Check sheet for the modelled part. Datum: model origin and axes. Units: mm. A direction names the side the tool comes from. Coordinates: 2 decimals unless noted, no trailing zeros. Loops run counter-clockwise (first coordinate to the right, second up) from the corner with the lowest first, then second, coordinate; pieces in that order, holes last. Notation, with made-up numbers: M -29,66 L 16,66 A33 ccw 16,104 Z; hole C 6,-7.5 d11. An arc over 180 degrees is marked long. Return JSON: item names as keys, results as strings.
from build123d import *

# Parameters (mm, degrees)
SKETCH1_W                = 63
SKETCH1_H                = 53
BOSS_EXTRUDE1_DEPTH      = 2
SKETCH2_W                = 15.24
SKETCH2_H                = 10.16
CUT_EXTRUDE1_DEPTH       = 1
BOSS_EXTRUDE2_DEPTH      = 0.1
BOSS_EXTRUDE2_DEPTH_BACK = 2.1
SKETCH4_R                = 2
SKETCH4_R_2              = 1
SKETCH4_W                = 5.013644296
SKETCH4_H                = 5.037668264
SKETCH4_W_2              = 4.110148076
SKETCH4_H_2              = 4.160405132
CUT_EXTRUDE2_START       = -2
SKETCH5_R                = 1
CUT_EXTRUDE2_DEPTH       = 2
EXTRUDE_THIN1_DEPTH      = 0.5
EXTRUDE_THIN1_DEPTH_BACK = 0.5
FILLET1_R                = 0.25


with BuildPart() as part:
    # Sketch1 → Boss-Extrude1 (new body)
    with BuildSketch(Plane.XY):
        with Locations((31.5, 26.5)):
            Rectangle(SKETCH1_W, SKETCH1_H)
    extrude(amount=-BOSS_EXTRUDE1_DEPTH)

    # Sketch2 → Cut-Extrude1 (cut)
    with BuildSketch(Plane.XY):
        Polygon((63, 26.54), (47.76, 26.54), (47.76, 36.7), (63, 36.66), align=None)
        with Locations((55.38, 41.82)):
            Rectangle(SKETCH2_W, SKETCH2_H)
        with Locations((55.38, 11.18)):
            Rectangle(SKETCH2_W, SKETCH2_H)
        Polygon((47.76, 16.3), (63, 16.34), (63, 26.46), (47.76, 26.46), align=None)
    extrude(amount=-CUT_EXTRUDE1_DEPTH, mode=Mode.SUBTRACT)

    # Sketch4 → Boss-Extrude2 (add, two sides: drawn at the far end of the back side and taken through both)
    # profile 1 of 3: a face of its own
    with BuildSketch(Plane.XY.offset(-BOSS_EXTRUDE2_DEPTH_BACK)):
        with Locations(Location((43.460589495, 50.19467241, 0), (0, 0, 180))):
            Circle(SKETCH4_R)
        with Locations(Location((43.460589495, 50.19467241, 0), (0, 0, 180))):
            Circle(SKETCH4_R_2, mode=Mode.SUBTRACT)
    # profile 2 of 3: a face of its own
    with BuildSketch(Plane.XY.offset(-BOSS_EXTRUDE2_DEPTH_BACK)):
        with Locations((60.493177852, 2.518834132)):
            Rectangle(SKETCH4_W, SKETCH4_H)
        with Locations(Location((60.493177852, 2.518834132, 0), (0, 0, 180))):
            Circle(SKETCH4_R_2, mode=Mode.SUBTRACT)
    # profile 3 of 3: a face of its own
    with BuildSketch(Plane.XY.offset(-BOSS_EXTRUDE2_DEPTH_BACK)):
        with Locations((60.041429742, 50.19467241)):
            Rectangle(SKETCH4_W_2, SKETCH4_H_2)
        with Locations(Location((60.041429742, 50.19467241, 0), (0, 0, 180))):
            Circle(SKETCH4_R_2, mode=Mode.SUBTRACT)
    extrude(amount=BOSS_EXTRUDE2_DEPTH + BOSS_EXTRUDE2_DEPTH_BACK)

    # Sketch5 → Cut-Extrude2 (cut)
    with BuildSketch(Plane.XY.offset(CUT_EXTRUDE2_START)):
        with Locations((60.493177852, 2.518834132)):
            Circle(SKETCH5_R)
        with Locations((60.041429742, 50.19467241)):
            Circle(SKETCH5_R)
        with Locations((43.460589495, 50.19467241)):
            Circle(SKETCH5_R)
    extrude(amount=CUT_EXTRUDE2_DEPTH, mode=Mode.SUBTRACT)

    # Sketch6 → Extrude-Thin1 (add, two sides: drawn at the far end of the back side and taken through both)
    with BuildSketch(Plane(origin=(0, 3, 0), x_dir=(-1, 0, 0), z_dir=(0, -1, 0)).offset(-EXTRUDE_THIN1_DEPTH_BACK)):
        with BuildLine():
            Line((-45.458769881, 0.670572303), (-45.458769881, -0.900340835))
            ThreePointArc((-45.458769881, -0.900340835), (-45.605216491, -1.253894226), (-45.958769881, -1.400340835))
            Line((-45.958769881, -1.400340835), (-52.153437165, -1.400340835))
            ThreePointArc((-52.153437165, -1.400340835), (-52.506990556, -1.253894226), (-52.653437165, -0.900340835))
            Line((-52.653437165, -0.900340835), (-52.653437165, 0.670572303))
            Line((-52.653437165, 0.670572303), (-53.153437165, 0.670572303))
            Line((-53.153437165, 0.670572303), (-53.153437165, -0.900340835))
            ThreePointArc((-53.153437165, -0.900340835), (-52.860543946, -1.607447616), (-52.153437165, -1.900340835))
            Line((-52.153437165, -1.900340835), (-45.958769881, -1.900340835))
            ThreePointArc((-45.958769881, -1.900340835), (-45.2516631, -1.607447616), (-44.958769881, -0.900340835))
            Line((-44.958769881, -0.900340835), (-44.958769881, 0.670572303))
            Line((-44.958769881, 0.670572303), (-45.458769881, 0.670572303))
        make_face()
    extrude(amount=EXTRUDE_THIN1_DEPTH + EXTRUDE_THIN1_DEPTH_BACK)

    # Fillet1
    fillet1_edges = [part.edges().sort_by_distance(p)[0] for p in [
        (45.458769881, 3.5, 0.450170417),
        (45.605216491, 3.5, 1.253894226),
        (52.653437165, 3.5, 0.450170417),
        (52.506990556, 3.5, 1.253894226),
        (45.458769881, 2.5, 0.450170417),
        (45.605216491, 2.5, 1.253894226),
        (52.653437165, 2.5, 0.450170417),
        (52.506990556, 2.5, 1.253894226),
        (44.958769881, 3.5, 0.450170417),
        (45.2516631, 3.5, 1.607447616),
        (53.153437165, 3.5, 0.450170417),
        (52.860543946, 3.5, 1.607447616),
        (44.958769881, 2.5, 0.450170417),
        (53.153437165, 2.5, 0.450170417),
        (52.860543946, 2.5, 1.607447616),
        (49.056103523, 2.5, 1.900340835),
        (49.056103523, 3.5, 1.400340835),
        (49.056103523, 2.5, 1.400340835),
        (49.056103523, 3.5, 1.900340835),
        (45.2516631, 2.5, 1.607447616),
    ]]
    fillet(fillet1_edges, radius=FILLET1_R - 0.0001)  # a hair under: the kernel refuses the full size


solid = part.part
1) Scan lines: line 1 along Z through (x, y) = (20, 50); line 2 along X through (y, z) = (37, -0.75). Record each from-to range of solid material in increasing order. Write a range as [from, to].
Answers:
{"line 1": "[-2, 0]", "line 2": "[0, 47.76]"}
2) Set-up check for faces 1 (the face through (59, 3, 0.1)), 2 (the face through (31, 53, -1)), 3 (the face through (55, 42, -1)): record each of +Z, -Z, +X, -X, +Y, -Y from which the full face is reachable in a straight line by a thin tool's end or side.
Answers:
{"face 1": "+Z, +X, +Y, -Y", "face 2": "+Z, -Z, +X, -X, +Y", "face 3": "+Z, +X"}
3) Section check A-A on y = 24. Record the cut outline in (x, z).
Answers:
{"outline": "M 0,-2 L 63,-2 L 63,-1 L 47.76,-1 L 47.76,0 L 0,0 Z"}
4) Section check C-C on x = 14.5. Record the cut outline in (y, z).
Answers:
{"outline": "M 0,-2 L 53,-2 L 53,0 L 0,0 Z"}
5) Go/stop test with flat-tipped pins: pin 1 Ø16 at (x, y) = (38, 22) entering from +Z; pin 2 Ø2.5 at (x, y) = (60.04, 50.19) entering from +Z; pin 3 Ø6 at (x, y) = (50.5, 16.5) entering from -Z. Record where each tip stops, or that it passes through.
Answers:
{"pin 1": "z = 0", "pin 2": "z = 0.1", "pin 3": "z = -2"}
6) Draft check along X on faces 4 (the face through (63, 26.1, -1.5)), 5 (the face through (0, 26, -1)), 6 (the face through (43, 49, 0.1)). Enter one of: +X half, -X half, draft (parallel to the pull), parting line (faces both ways), or undercut.
Answers:
{"face 4": "+X half", "face 5": "-X half", "face 6": "draft"}
7) Section check B-B on x = 57. Record the cut outline in (y, z).
Answers:
{"outline": "M 0,-2 L 53,-2 L 53,0 L 46.9,0 L 46.9,-1 L 36.74,-1 L 36.74,0 L 36.68,0 L 36.68,-1 L 26.54,-1 L 26.54,0 L 26.46,0 L 26.46,-1 L 16.32,-1 L 16.32,0 L 16.26,0 L 16.26,-1 L 6.1,-1 L 6.1,0 L 0,0 Z"}
